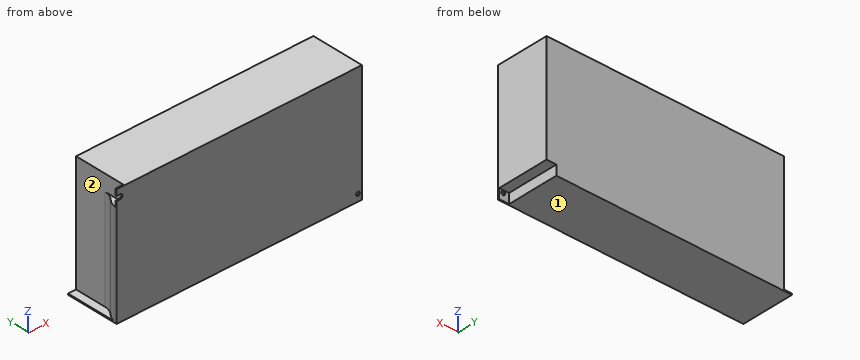
```python
from build123d import *

# Parameters (mm, degrees)
SKETCH1_W           = 200
SKETCH1_H           = 97
BOSS_EXTRUDE1_DEPTH = 43
CUT_EXTRUDE1_DEPTH  = 96
SKETCH3_W           = 6.5
SKETCH3_H           = 13
SKETCH3_W_2         = 8
SKETCH3_H_2         = 8
CUT_EXTRUDE2_DEPTH  = 42
SKETCH4_R           = 1.6
CUT_EXTRUDE3_DEPTH  = 119.811826011


with BuildPart() as part:
    # Sketch1 → Boss-Extrude1 (new body)
    with BuildSketch(Plane(origin=(0, 0, 0), x_dir=(1, 0, 0), z_dir=(0, 1, 0))):
        Rectangle(SKETCH1_W, SKETCH1_H)
    extrude(amount=BOSS_EXTRUDE1_DEPTH)

    # Sketch2 → Cut-Extrude1 (cut)
    with BuildSketch(Plane.XY.offset(48.5)):
        with BuildLine():
            Line((-93.5, 43), (-93.5, 17.5))
            ThreePointArc((-93.5, 17.5), (-94.365227926, 12.762263764), (-96.84920953, 8.636176103))
            ThreePointArc((-96.84920953, 8.636176103), (-98.879103447, 5.571249802), (-100, 2.070130916))
            Line((-100, 2.070130916), (-100, 43))
            Line((-100, 43), (-93.5, 43))
        make_face()
    extrude(amount=-CUT_EXTRUDE1_DEPTH, mode=Mode.SUBTRACT)

    # Sketch3 → Cut-Extrude2 (cut)
    with BuildSketch(Plane(origin=(0, 43, 0), x_dir=(1, 0, 0), z_dir=(0, 1, 0))):
        with Locations((-96.75, -42)):
            Rectangle(SKETCH3_W, SKETCH3_H)
        with Locations((96, 44.5)):
            Rectangle(SKETCH3_W_2, SKETCH3_H_2)
    extrude(amount=-CUT_EXTRUDE2_DEPTH, mode=Mode.SUBTRACT)

    # Sketch4 → Cut-Extrude3 (cut, through all)
    with BuildSketch(Plane(origin=(0, 1, 0), x_dir=(1, 0, 0), z_dir=(0, 1, 0))):
        with Locations(Location((96.8, 42.7, 0), (0, 0, 270))):
            Circle(SKETCH4_R)
        with BuildLine():
            Line((-97.001938149, -43.7), (-106.165293612, -43.7))
            ThreePointArc((-106.165293612, -43.7), (-108.065293612, -41.8), (-106.165293612, -39.9))
            Line((-106.165293612, -39.9), (-97.001938149, -39.9))
            ThreePointArc((-97.001938149, -39.9), (-95.101938149, -41.8), (-97.001938149, -43.7))
        make_face()
    extrude(amount=-CUT_EXTRUDE3_DEPTH, mode=Mode.SUBTRACT)


solid = part.part
```
Design review of the part built by this model. Coordinates are the model's own, in mm. Face numbers are marked on the shaded views. A direction names the side the tool comes from. Round coordinates to 2 decimals unless told otherwise and drop trailing zeros. Write each loop counter-clockwise with the first axis right and the second up, starting at its lowest first coordinate (ties: lowest second). Pieces come first, ordered by that corner, then holes.
Item 1: We need section A-A on y = 34. Write out the cut boundary in (x, z).
Item 2: We need section C-C on z = 31. Write out the cut boundary in (x, y), and give its area (3 significant figures).
Item 3: For the marked faces 1 and 2, list the 3-axis set-ups (+Z, -Z, +X, -X, +Y, -Y) from which the entire face can be reached by the end or side of a thin tool; tool diameter is ignored.
Item 4: Clearance check with flat-ended pins moving along their axes: pin 1 Ø12.5 at (y, z) = (21, -1.5) entering from -X; pin 2 Ø8 at (y, z) = (15.5, 26.5) entering from -X; pin 3 Ø6 at (y, z) = (21, -17.5) entering from -X; pin 4 Ø3 at (x, z) = (96.8, -42.7) entering from -Y. State where each tip first meets the part, or that it passes through.
Item 5: For probe 1 along Z at (x, y) = (96.8, 0.55); probe 2 along X at (y, z) = (0.45, -42.7); probe 3 along X at (y, z) = (27, -18), list the stretches that pass through material, from the lowest coordinate up.
Item 6: We need section B-B on z = 41.8. Write out the cut boundary in (x, y), and give its area (3 significant figures).
Returned:
1. outline: (-100, -48.5) - (92, -48.5) - (92, -40.5) - (100, -40.5) - (100, 48.5) - (-93.5, 48.5) - (-93.5, -47.5) - (-100, -47.5) - close
2. outline: (-100, 0) - (100, 0) - (100, 43) - (-93.5, 43) - (-93.5, 17.5) arc R13.4 cw to (-96.85, 8.64) arc R13.4 ccw to (-100, 2.07) - close
2. area: 8,380 mm2
3. face 1: -Z, +X, -X, +Y, -Y
3. face 2: +Z, -X, +Y
4. pin 1: stops at x = -93.79
4. pin 2: stops at x = -94.92
4. pin 3: stops at x = -93.5
4. pin 4: passes through
5. probe 1: z = -48.5 to -44.3, -41.1 to 48.5
5. probe 2: x = -100 to 95.2, 98.4 to 100
5. probe 3: x = -93.5 to 100
6. outline: (-95.1, 0) - (100, 0) - (100, 43) - (-93.5, 43) - (-93.5, 1) - (-95.1, 1) - close
6. area: 8,320 mm2
